```python
from build123d import *

# Parameters (mm, degrees)
F0_W      = 50.6787924096
F0_H      = 103.9609350264
F1_DEPTH  = 25.4
F4_W      = 18.917764537
F4_H      = 103.9609350264
F5_DEPTH  = 25.4
F6_W      = 19.2797044292
F6_H      = 103.9609350264
F7_DEPTH  = 25.4
F10_W     = 25.2526141703
F10_H     = 25.1658372581
F11_DEPTH = 2.54
F28_W     = 19.1976749338
F28_H     = 18.704187125
F29_DEPTH = 1.27
F30_W     = 19.0913220868
F30_H     = 18.744206056
F31_DEPTH = 1.27
F32_W     = 25.4
F32_H     = 25.8600655943
F32_W_2   = 19.0913220868
F32_H_2   = 18.744206056
F33_DEPTH = 2.54


# Not quite as in the source:
# - the program builds the solid bodies; features that only make, move or delete a surface that nothing else refers to are left out


with BuildPart() as f1:
    # F0 (on Front) → F1 (new body)
    with BuildSketch(Plane.XZ):
        with Locations((1.8223566003, -0.2603363246)):
            Rectangle(F0_W, F0_H)
    extrude(amount=F1_DEPTH)

    # F4 (on face) → F5 (join)
    with BuildSketch(Plane.XZ.offset(25.4)):
        with Locations((0.5206721835, -0.2603363246)):
            Rectangle(F4_W, F4_H)
    extrude(amount=F5_DEPTH)

    # F6 (on face) → F7 (join)
    with BuildSketch(Plane(origin=(0, 0, 0), x_dir=(-1, 0, 0), z_dir=(0, 1, 0))):
        with Locations((-1.1341772042, -0.2603363246)):
            Rectangle(F6_W, F6_H)
    extrude(amount=F7_DEPTH)

    # F9: sweep along a path in F8
    with BuildLine(Plane.XY.offset(51.7201311886)) as f9_path:
        Line((-23.5170396045, -12.7), (27.1617528051, -12.7))
    # F3 (on face) → F9 (sweep)
    with BuildSketch(Plane(origin=(-23.5170396045, 0, 0), x_dir=(0, -1, 0), z_dir=(-1, 0, 0))):
        with BuildLine():
            Line((0, 51.7201311886), (25.4, 51.7201311886))
            ThreePointArc((25.4, 51.7201311886), (12.7, 64.4201311886), (0, 51.7201311886))
        make_face()
    sweep(path=f9_path.line)

    # F10 (on face) → F11 (join)
    with BuildSketch(Plane.YZ.offset(27.1617528051)):
        with Locations((-12.6263070852, 38.9636550099)):
            Rectangle(F10_W, F10_H)
    extrude(amount=F11_DEPTH)

    # F28 (on face) → F29 (cut)
    with BuildSketch(Plane.YZ.offset(29.7017528051)):
        with Locations((-12.9288590979, 38.9715339988)):
            Rectangle(F28_W, F28_H)
    extrude(amount=-F29_DEPTH, mode=Mode.SUBTRACT)

    # F30 (on face) → F31 (cut)
    with BuildSketch(Plane(origin=(-23.5170396045, 0, 0), x_dir=(0, -1, 0), z_dir=(-1, 0, 0))):
        with Locations((12.9300323315, 38.8768771663)):
            Rectangle(F30_W, F30_H)
    extrude(amount=-F31_DEPTH, mode=Mode.SUBTRACT)

    # F32 (on face) → F33 (join)
    with BuildSketch(Plane(origin=(-23.5170396045, 0, 0), x_dir=(0, -1, 0), z_dir=(-1, 0, 0))):
        with Locations((12.7, 38.7900983915)):
            Rectangle(F32_W, F32_H)
        with Locations((12.9300323315, 38.8768771663)):
            Rectangle(F32_W_2, F32_H_2, mode=Mode.SUBTRACT)
    extrude(amount=F33_DEPTH)


solid = f1.part
```
The listing builds one solid part. Answer for the finished solid, in the listing's coordinates (mm). A direction names the side the tool comes from. Round coordinates to 2 decimals unless told otherwise and drop trailing zeros. Loops run counter-clockwise (first coordinate to the right, second up) from the corner with the lowest first, then second, coordinate; pieces in that order, holes last.
Q1. For a pull along Z with two mould halves and no side action, classify faces 6 (the face through (-24, -3.384, 39)), 7 (the face through (1, 13, 51.72)), 8 (the face through (-24, -13, 48.249)), 9 (the face through (28, -13, 26.381)) as released by +Z, released by -Z, zero draft, split by the parting line, or undercut.
Q2. Given pin 1 Ø12.5 at (y, z) = (-14.5, 0) entering from -X; pin 2 Ø20.5 at (y, z) = (13, -3.5) entering from -X; pin 3 Ø12 at (x, z) = (17, 14) entering from +Y, each flat-ended and moving along its own axis, determine where each tip first touches the part or whether it passes through.
Q3. Which of the six approach directions +Z, -Z, +X, -X, +Y, -Y give full straight-line access (tool end or side, diameter ignored) to faces 1 (the face through (-24, -13, 29.505)), 2 (the face through (18, -25.4, 0)), 3 (the face through (28, -13, 51.547)), 4 (the face through (-8.938, -38, -1)), 5 (the face through (-17, 0, -1))?
Q4. Section C-C, the plane x = -2.5 is taken. Determine the outline of the cut face in (y, z), then the cut area to 3 significant figures.
Q5. Section A-A, the plane z = 18 is taken. Determine the outline of the cut face in (x, y), then the cut area to 3 significant figures.
Q6. Section B-B, the plane y = -12.7 is taken. Determine the outline of the cut face in (x, z).
Q7. Find the intervals of material crossed by line 1 (Z direction, x = 9.5, y = -35); line 2 (X direction, y = -35, z = -47); line 3 (Y direction, x = 10.5, z = -31), in increasing order.
Q8. Section D-D, the plane z = 38 is taken. Determine the outline of the cut face in (x, y).
Completed:
1. face 6: undercut
1. face 7: released by +Z
1. face 8: undercut
1. face 9: released by -Z
2. pin 1: stops at x = -23.52
2. pin 2: stops at x = -8.51
2. pin 3: stops at y = 0
3. face 1: -X
3. face 2: +Z, -Z, +X, -Y
3. face 3: +Z, +X, +Y, -Y
3. face 4: +Z, -Z, -X, -Y
3. face 5: +Z, -Z, -X, +Y
4. outline: (-50.8, -52.24) - (25.4, -52.24) - (25.4, 51.72) - (0, 51.72) arc R12.7 ccw to (-25.4, 51.72) - (-50.8, 51.72) - close
4. area: 8,180 mm2
5. outline: (-23.52, -25.4) - (-8.94, -25.4) - (-8.94, -50.8) - (9.98, -50.8) - (9.98, -25.4) - (27.16, -25.4) - (27.16, 0) - (10.77, 0) - (10.77, 25.4) - (-8.51, 25.4) - (-8.51, 0) - (-23.52, 0) - close
5. area: 2,260 mm2
6. outline: (-26.06, 25.86) - (-23.52, 25.86) - (-23.52, -52.24) - (27.16, -52.24) - (27.16, 26.38) - (29.7, 26.38) - (29.7, 29.62) - (28.43, 29.62) - (28.43, 48.32) - (29.7, 48.32) - (29.7, 51.55) - (27.16, 51.55) - (27.16, 64.42) - (-23.52, 64.42) - (-23.52, 51.72) - (-26.06, 51.72) - (-26.06, 48.25) - (-22.25, 48.25) - (-22.25, 29.5) - (-26.06, 29.5) - close
7. line 1: z = -52.24 to 51.72
7. line 2: x = -8.94 to 9.98
7. line 3: y = -25.4 to 25.4
8. outline: (-26.06, -25.4) - (-8.94, -25.4) - (-8.94, -50.8) - (9.98, -50.8) - (9.98, -25.4) - (27.16, -25.4) - (27.16, -25.25) - (29.7, -25.25) - (29.7, -22.53) - (28.43, -22.53) - (28.43, -3.33) - (29.7, -3.33) - (29.7, 0) - (10.77, 0) - (10.77, 25.4) - (-8.51, 25.4) - (-8.51, 0) - (-26.06, 0) - (-26.06, -3.38) - (-22.25, -3.38) - (-22.25, -22.48) - (-26.06, -22.48) - close
